CAD build for the part. Positions are in the model's coordinates, mm. Coordinates: 2 decimals unless noted, no trailing zeros. Write each question's results on one line, items separated by ' | '. Start each with the question number.
Q1. Wall check: probe 1 along Y at (x, z) = (8, 771); probe 2 along Y at (x, z) = (2.5, 179); probe 3 along X at (y, z) = (-7.25, 738.5). Give the ranges that are in metal, low to high.
Q2. Band-saw the part on A-A, the plane z = 520.5. Count the separate pieces of the cut face and the enclosed holes in it, then the cut area to 3 significant figures.
Q3. Pin check, flat tips, straight feed: P1, Ø2, axis at y = -1, z = 613, coming from the -X side; P2, Ø1.4, axis at x = 0, z = 563.5, coming from the -Y side; P3, Ø1.4, axis at x = 0, z = 708, coming from the +Y side. Stop position of each tip, or through.
```python
from build123d import *

# Parameters (mm, degrees)
SKETCH_1_R      = 1.65
SKETCH_1_R_2    = 1.75
EXTRUDE_1_DEPTH = 1000


with BuildPart() as part:
    # 草图1 → 凸台-拉伸1 (new body)
    with BuildSketch(Plane.XY):
        Polygon((-2.177197952, 9.242987377), (-9.877197952, 9.242987377), (-9.877197952, 1.542987377), (-8.377197952, 1.542987377), (-8.377197952, 3.492987377), (-4.677197952, 3.492987377), (-4.677197952, 1.542987377), (-2.777197952, 1.542987377), (-2.777197952, -3.057012623), (-4.677197952, -3.057012623), (-4.677197952, -5.007012623), (-8.377197952, -5.007012623), (-8.377197952, -3.057012623), (-9.877197952, -3.057012623), (-9.877197952, -10.757012623), (-2.177197952, -10.757012623), (-2.177197952, -9.257012623), (-4.127197952, -9.257012623), (-4.127197952, -5.557012623), (-2.177197952, -5.557012623), (-2.177197952, -3.657012623), (2.422802048, -3.657012623), (2.422802048, -5.557012623), (4.372802048, -5.557012623), (4.372802048, -9.257012623), (2.422802048, -9.257012623), (2.422802048, -10.757012623), (10.122802048, -10.757012623), (10.122802048, -3.057012623), (8.622802048, -3.057012623), (8.622802048, -5.007012623), (4.922802048, -5.007012623), (4.922802048, -3.057012623), (3.022802048, -3.057012623), (3.022802048, 1.542987377), (4.922802048, 1.542987377), (4.922802048, 3.492987377), (8.622802048, 3.492987377), (8.622802048, 1.542987377), (10.122802048, 1.542987377), (10.122802048, 9.242987377), (2.422802048, 9.242987377), (2.422802048, 7.742987377), (4.372802048, 7.742987377), (4.372802048, 4.042987377), (2.422802048, 4.042987377), (2.422802048, 2.142987377), (-2.177197952, 2.142987377), (-2.177197952, 4.042987377), (-4.127197952, 4.042987377), (-4.127197952, 7.742987377), (-2.177197952, 7.742987377), align=None)
        with Locations((0.122802048, -0.757012623)):
            Circle(SKETCH_1_R, mode=Mode.SUBTRACT)
        with Locations((-7.002197952, 6.367987377)):
            Circle(SKETCH_1_R_2, mode=Mode.SUBTRACT)
        with Locations((7.247802048, 6.367987377)):
            Circle(SKETCH_1_R_2, mode=Mode.SUBTRACT)
        with Locations((-7.002197952, -7.882012623)):
            Circle(SKETCH_1_R_2, mode=Mode.SUBTRACT)
        with Locations((7.247802048, -7.882012623)):
            Circle(SKETCH_1_R_2, mode=Mode.SUBTRACT)
    extrude(amount=EXTRUDE_1_DEPTH)


solid = part.part
```
Results below:
1) probe 1: y = -10.76 to -9.46, -6.3 to -5.01, 3.49 to 4.79, 7.95 to 9.24 | probe 2: y = -10.76 to -9.26, -5.56 to 4.04, 7.74 to 9.24 | probe 3: x = -9.88 to -8.63, -5.37 to -4.13, 4.37 to 5.62, 8.88 to 10.12
2) separate pieces: 1 | enclosed holes: 5 | area: 165 mm²
3) P1: stops at x = -2.78 | P2: stops at y = -3.66 | P3: stops at y = 2.14
